from build123d import *

# Parameters (mm, degrees)
F0_W      = 43.18
F0_H      = 21.971
F0_W_2    = 40.64
F0_H_2    = 19.431
F1_DEPTH  = 16.1544
F0_W_3    = 37.592
F0_H_3    = 16.383
F2_DEPTH  = 1.27
F3_R      = 1.27
F4_R      = 1.27
F5_R      = 1.785938
F6_DEPTH  = 7.62
F7_R      = 1.785938
F8_DEPTH  = 7.62
F9_W      = 1.27
F9_H      = 5.068467
F10_DEPTH = 3.05
F12_DEPTH = 5.08
F14_DEPTH = 5.08


with BuildPart() as f1:
    # F0 (on Front) → F1 (new body)
    with BuildSketch(Plane.XZ):
        Rectangle(F0_W, F0_H)
        Rectangle(F0_W_2, F0_H_2, mode=Mode.SUBTRACT)
    extrude(amount=F1_DEPTH)

    # F0 (on Front) → F2 (join)
    with BuildSketch(Plane.XZ):
        Rectangle(F0_W_2, F0_H_2)
        Rectangle(F0_W_3, F0_H_3, mode=Mode.SUBTRACT)
    extrude(amount=F2_DEPTH)

    # F3
    f3_edges = [f1.edges().sort_by_distance(p)[0] for p in [
        (-21.59, -8.0772, 10.9855),
        (-21.59, -8.0772, -10.9855),
        (21.59, -8.0772, -10.9855),
        (21.59, -8.0772, 10.9855),
    ]]
    fillet(f3_edges, radius=F3_R)

    # F4
    f4_edges = [f1.edges().sort_by_distance(p)[0] for p in [
        (0, 0, -10.9855),
    ]]
    fillet(f4_edges, radius=F4_R)

    # F5 (on face) → F6 (cut)
    with BuildSketch(Plane.YZ.offset(21.59)):
        with Locations((-8.7122, 0)):
            Circle(F5_R)
    extrude(amount=-F6_DEPTH, mode=Mode.SUBTRACT)

    # F7 (on face) → F8 (cut)
    with BuildSketch(Plane(origin=(-21.59, 0, 0), x_dir=(0, -1, 0), z_dir=(-1, 0, 0))):
        with Locations((8.7122, 0)):
            Circle(F7_R)
    extrude(amount=-F8_DEPTH, mode=Mode.SUBTRACT)

    # F9 (on face) → F10 (join)
    with BuildSketch(Plane.XZ.offset(16.1544)):
        with Locations((-20.955, -0.002476)):
            Rectangle(F9_W, F9_H)
        with Locations((20.955, -0.002476)):
            Rectangle(F9_W, F9_H)
    extrude(amount=F10_DEPTH)

    # F11 (on face) → F12 (join)
    with BuildSketch(Plane(origin=(0, 0, -2.53671), x_dir=(1, 0, 0), z_dir=(0, 0, -1))):
        with BuildLine():
            Line((20.32, 22.2044), (20.32, 19.2044))
            Line((20.32, 19.2044), (21.59, 19.2044))
            Line((21.59, 19.2044), (22.479, 19.2044))
            Line((22.479, 19.2044), (21.859416, 21.295234))
            ThreePointArc((21.859416, 21.295234), (21.401571, 21.952034), (20.641755, 22.2044))
            Line((20.641755, 22.2044), (20.32, 22.2044))
        make_face()
    extrude(amount=-F12_DEPTH)

    # F13 (on face) → F14 (join)
    with BuildSketch(Plane(origin=(0, 0, -2.53671), x_dir=(1, 0, 0), z_dir=(0, 0, -1))):
        with BuildLine():
            Line((-21.59, 19.2044), (-20.32, 19.2044))
            Line((-20.32, 19.2044), (-20.32, 22.46322))
            Line((-20.32, 22.46322), (-20.614604, 22.46322))
            ThreePointArc((-20.614604, 22.46322), (-21.384353, 22.203362), (-21.839101, 21.530127))
            Line((-21.839101, 21.530127), (-22.479, 19.2044))
            Line((-22.479, 19.2044), (-21.59, 19.2044))
        make_face()
    extrude(amount=-F14_DEPTH)


solid = f1.part
For this review, take the finished solid that the model builds, in its own axes (mm). A direction names the side the tool comes from. Round coordinates to 2 decimals unless told otherwise and drop trailing zeros. Loops run counter-clockwise (first coordinate to the right, second up) from the corner with the lowest first, then second, coordinate; pieces in that order, holes last. Notation, with made-up numbers: (-39.75, 32) - (11.25, 32) arc R33 ccw to (11.25, 63) - close; hole circle Ø10 at (-37.75, 35). An arc over 180 degrees is marked (long way). One line per item, written item: value. Start each with the question number.
Item 1: Clearance check with flat-ended pins moving along their axes: pin 1 Ø1.1 at (x, z) = (21.5, 1) entering from +Y; pin 2 Ø3 at (y, z) = (-12.5, -5.5) entering from -X; pin 3 Ø0.6 at (x, y) = (-21.5, -21) entering from -Z; pin 4 Ø1.4 at (x, y) = (8, -1) entering from -Z. State where each tip first meets the part, or that it passes through.
Item 2: Take a section at D-D (y = -9). Give the boundary of the cut face in (x, z), plus the area to 3 significant figures.
Item 3: Take a section at B-B (z = -4.75). Give the boundary of the cut face in (x, y), plus the area to 3 significant figures.
Item 4: For L1, parallel to Z at x = -4, y = -15; L2, parallel to X at y = -13.5, z = 6.5; L3, parallel to Y at x = -4.5, z = -8.5, list the stretches that pass through material, from the lowest coordinate up.
Item 5: For faces 4 (the flat face through (21.59, -10, -2)), 5 (the flat face through (-2, -1.27, -9)), 6 (the flat face through (21, -21, -2.537)), 7 (the flat face through (21, -21, 2.543)), 8 (the cylindrical face through (-21.23, -8.82, 10.6)), list the 3-axis set-ups (+Z, -Z, +X, -X, +Y, -Y) from which the entire face can be reached by the end or side of a thin tool; tool diameter is ignored.
Item 6: Take a section at A-A (z = 0). Give the boundary of the cut face in (x, y).
Item 7: Take a section at C-C (x = 5.5). Give the boundary of the cut face in (y, z).
Item 8: The part is to be moulded in two halves that separate along Y. For faces 1 (the cylindrical face through (-0.28, -0.36, 10.6)), 2 (the cylindrical face through (-21.23, -8.82, -10.6)), 3 (the cylindrical face through (-20.96, -6.93, 0.08)), say which applies: +Y half, -Y half, draft (parallel to the pull), parting line (faces both ways), or undercut.
Answer below:
1. pin 1: stops at y = -0.17
1. pin 2: stops at x = -21.59
1. pin 3: stops at z = -2.54
1. pin 4: stops at z = -10.99
2. outline: (-21.59, -9.72) arc R1.27 ccw to (-20.32, -10.99) - (20.32, -10.99) arc R1.27 ccw to (21.59, -9.72) - (21.59, -1.76) - (20.32, -1.76) - (20.32, -9.72) - (-20.32, -9.72) - (-20.32, -1.76) - (-21.59, -1.76) - close; (-21.59, 1.76) - (-20.32, 1.76) - (-20.32, 9.72) - (20.32, 9.72) - (20.32, 1.76) - (21.59, 1.76) - (21.59, 9.72) arc R1.27 ccw to (20.32, 10.99) - (-20.32, 10.99) arc R1.27 ccw to (-21.59, 9.72) - close
2. area: 149 mm2
3. outline: (-21.59, -16.15) - (-20.32, -16.15) - (-20.32, -1.27) - (-18.8, -1.27) - (-18.8, 0) - (-20.32, 0) arc R1.27 ccw to (-21.59, -1.27) - close; (18.8, -1.27) - (20.32, -1.27) - (20.32, -16.15) - (21.59, -16.15) - (21.59, -1.27) arc R1.27 ccw to (20.32, 0) - (18.8, 0) - close
3. area: 44.2 mm2
4. L1: z = -10.99 to -9.72, 9.72 to 10.99
4. L2: x = -21.59 to -20.32, 20.32 to 21.59
4. L3: y = -1.27 to 0
5. face 4: +Z, -Z, +X, +Y
5. face 5: -Y
5. face 6: -Z, +X, -X, -Y
5. face 7: +Z, +X, -X, -Y
5. face 8: +Z, -X, +Y, -Y
6. outline: (-22.48, -19.2) - (-21.84, -21.53) arc R1.27 ccw to (-20.61, -22.46) - (-20.32, -22.46) - (-20.32, -10.5) - (-21.59, -10.5) - (-21.59, -19.2) - close; (-21.59, -6.93) - (-20.32, -6.93) - (-20.32, -1.27) - (-18.8, -1.27) - (-18.8, 0) - (-20.32, 0) arc R1.27 ccw to (-21.59, -1.27) - close; (18.8, -1.27) - (20.32, -1.27) - (20.32, -6.93) - (21.59, -6.93) - (21.59, -1.27) arc R1.27 ccw to (20.32, 0) - (18.8, 0) - close; (20.32, -22.2) - (20.64, -22.2) arc R1.27 ccw to (21.86, -21.3) - (22.48, -19.2) - (21.59, -19.2) - (21.59, -10.5) - (20.32, -10.5) - close
7. outline: (-16.15, -10.99) - (-1.27, -10.99) arc R1.27 ccw to (0, -9.72) - (0, -8.19) - (-1.27, -8.19) - (-1.27, -9.72) - (-16.15, -9.72) - close; (-16.15, 9.72) - (-1.27, 9.72) - (-1.27, 8.19) - (0, 8.19) - (0, 9.72) arc R1.27 ccw to (-1.27, 10.99) - (-16.15, 10.99) - close
8. face 1: +Y half
8. face 2: draft
8. face 3: undercut
